from build123d import *

# Parameters (mm, degrees)
SKETCH1_W            = 82.8
SKETCH1_H            = 327.3
PCB_EXTRUDE_DEPTH    = 1.6
SKETCH2_W            = 82.8
SKETCH2_H            = 327.3
SKETCH2_W_2          = 82.5
SKETCH2_H_2          = 327
OFFSET_EDGES_DEPTH   = 10
CORNER_FILLETS_R     = 1
SKETCH3_R            = 1.5
SKETCH3_W            = 15
SKETCH3_H            = 6
SOLAR_HOLE_DEPTH     = 169.630876473
SOLAR_HOLE_FILLET_R  = 0.5
M2_CLEARANCE_HOLE1_D = 2.6
SKETCH9_W            = 1.75
SKETCH9_H            = 2.6
CUT_EXTRUDE1_DEPTH   = 169.630876473
FILLET1_R            = 2.5


with BuildPart() as part:
    # Sketch1 → PCB extrude (new body)
    with BuildSketch(Plane.XY):
        Rectangle(SKETCH1_W, SKETCH1_H)
    extrude(amount=PCB_EXTRUDE_DEPTH)

    # Sketch2 → offset edges (cut)
    with BuildSketch(Plane.XY):
        Rectangle(SKETCH2_W, SKETCH2_H)
        Rectangle(SKETCH2_W_2, SKETCH2_H_2, mode=Mode.SUBTRACT)
    extrude(amount=OFFSET_EDGES_DEPTH, mode=Mode.SUBTRACT)

    # corner fillets
    corner_fillets_edges = [part.edges().sort_by_distance(p)[0] for p in [
        (41.25, 163.5, 0.8),
        (-41.25, 163.5, 0.8),
        (-41.25, -163.5, 0.8),
        (41.25, -163.5, 0.8),
    ]]
    fillet(corner_fillets_edges, radius=CORNER_FILLETS_R)

    # Sketch3 → Solar hole (cut, symmetric)
    with BuildSketch(Plane.XY):
        with Locations((0, 160.95)):
            Circle(SKETCH3_R)
        with BuildLine():
            Line((-2.999999999, 158.15), (2.999999999, 158.15))
            Line((2.999999999, 158.15), (2.999999999, 161.65))
            Line((2.999999999, 161.65), (9.5, 161.65))
            ThreePointArc((9.5, 161.65), (10, 161.15), (9.5, 160.65))
            Line((9.5, 160.65), (6.2, 160.65))
            Line((6.2, 160.65), (6.2, 153.35))
            Line((6.2, 153.35), (-6.2, 153.35))
            Line((-6.2, 153.35), (-6.2, 160.65))
            Line((-6.2, 160.65), (-9.5, 160.65))
            ThreePointArc((-9.5, 160.65), (-10, 161.15), (-9.5, 161.65))
            Line((-9.5, 161.65), (-2.999999999, 161.65))
            Line((-2.999999999, 161.65), (-2.999999999, 158.15))
        make_face()
        with Locations((0, 42.125)):
            Rectangle(SKETCH3_W, SKETCH3_H)
    solar_hole = extrude(amount=SOLAR_HOLE_DEPTH, both=True, mode=Mode.SUBTRACT)

    # Solar hole mirror: Solar hole across plane
    add(solar_hole.mirror(Plane.ZX), mode=Mode.SUBTRACT)

    # Solar Hole Fillet
    solar_hole_fillet_edges = [part.edges().sort_by_distance(p)[0] for p in [
        (2.999999999, 161.65, 0.8),
        (2.999999999, 158.15, 0.8),
        (-2.999999999, 158.15, 0.8),
        (-2.999999999, 161.65, 0.8),
        (-6.2, 160.65, 0.8),
        (-6.2, 153.35, 0.8),
        (6.2, 153.35, 0.8),
        (6.2, 160.65, 0.8),
        (6.2, -160.65, 0.8),
        (6.2, -153.35, 0.8),
        (-6.2, -153.35, 0.8),
        (-6.2, -160.65, 0.8),
        (-2.999999999, -161.65, 0.8),
        (-2.999999999, -158.15, 0.8),
        (2.999999999, -158.15, 0.8),
        (2.999999999, -161.65, 0.8),
    ]]
    fillet(solar_hole_fillet_edges, radius=SOLAR_HOLE_FILLET_R)

    # M2 Clearance Hole1 (through all)
    with Locations(Plane.XY.offset(1.6)):
        with Locations((-39.5, 143.75), (-39.5, 113.75), (-39.5, 83.75), (-39.5, 27.25), (-39.5, 0.75), (-39.5, -25.75), (-39.5, -83.75), (-39.5, -113.75), (-39.5, -143.75), (-16.5, -117.75), (16.5, -117.75), (39.5, -143.75), (39.5, -113.75), (39.5, -83.75), (16.5, -58.1), (-16.5, -58.1), (39.5, -25.75), (39.5, 0.75), (16.5, 0), (-16.5, 0), (39.5, 27.25), (16.5, 58.1), (-16.5, 58.1), (16.5, 117.75), (-16.5, 117.75), (39.5, 83.75), (39.5, 113.75), (39.5, 143.75)):
            Hole(M2_CLEARANCE_HOLE1_D / 2)

    # Sketch9 → Cut-Extrude1 (cut, through all)
    with BuildSketch(Plane.XY):
        with Locations((-40.375, 143.75)):
            Rectangle(SKETCH9_W, SKETCH9_H)
        with Locations((40.375, 143.75)):
            Rectangle(SKETCH9_W, SKETCH9_H)
        with Locations((40.375, 113.75)):
            Rectangle(SKETCH9_W, SKETCH9_H)
        with Locations((40.375, 83.75)):
            Rectangle(SKETCH9_W, SKETCH9_H)
        with Locations((-40.375, 113.75)):
            Rectangle(SKETCH9_W, SKETCH9_H)
        with Locations((-40.375, 83.75)):
            Rectangle(SKETCH9_W, SKETCH9_H)
        with Locations((40.375, 27.25)):
            Rectangle(SKETCH9_W, SKETCH9_H)
        with Locations((-40.375, 27.25)):
            Rectangle(SKETCH9_W, SKETCH9_H)
        with Locations((40.375, 0.75)):
            Rectangle(SKETCH9_W, SKETCH9_H)
        with Locations((-40.375, 0.75)):
            Rectangle(SKETCH9_W, SKETCH9_H)
        with Locations((40.375, -25.75)):
            Rectangle(SKETCH9_W, SKETCH9_H)
        with Locations((-40.375, -25.75)):
            Rectangle(SKETCH9_W, SKETCH9_H)
        with Locations((40.375, -83.75)):
            Rectangle(SKETCH9_W, SKETCH9_H)
        with Locations((-40.375, -83.75)):
            Rectangle(SKETCH9_W, SKETCH9_H)
        with Locations((40.375, -113.75)):
            Rectangle(SKETCH9_W, SKETCH9_H)
        with Locations((-40.375, -113.75)):
            Rectangle(SKETCH9_W, SKETCH9_H)
        with Locations((40.375, -143.75)):
            Rectangle(SKETCH9_W, SKETCH9_H)
        with Locations((-40.375, -143.75)):
            Rectangle(SKETCH9_W, SKETCH9_H)
    extrude(amount=CUT_EXTRUDE1_DEPTH, mode=Mode.SUBTRACT)

    # Fillet1
    fillet1_edges = [part.edges().sort_by_distance(p)[0] for p in [
        (-7.5, -39.125, 0.8),
        (-7.5, -45.125, 0.8),
        (7.5, -45.125, 0.8),
        (7.5, -39.125, 0.8),
        (-7.5, 45.125, 0.8),
        (-7.5, 39.125, 0.8),
        (7.5, 39.125, 0.8),
        (7.5, 45.125, 0.8),
    ]]
    fillet(fillet1_edges, radius=FILLET1_R)


solid = part.part
Source: CAD feature listing. Evaluate the final solid. Frame: model axes, mm. Give positions to 0.01 mm unless a question says otherwise; leave off trailing zeros. Answer as a JSON object with one key per item and string values.
Q1. Cut plane A-A, the plane z = 0.8. Count the separate pieces of the cut face and the enclosed holes in it, then the cut area to 3 significant figures.
Geometry check:
{"separate pieces": "1", "enclosed holes": "16", "area": "26,400 mm^2"}
Q2. Ray query, line 1 along Y through (x, z) = (-16.5, 1.15); line 2 along X through (y, z) = (117.75, 0.7); line 3 along X through (y, z) = (-144, 0.95). Return the intervals inside material, ascending.
Geometry check:
{"line 1": "y = -163.5 to -119.05, -116.45 to -59.4, -56.8 to -1.3, 1.3 to 56.8, 59.4 to 116.45, 119.05 to 163.5", "line 2": "x = -41.25 to -17.8, -15.2 to 15.2, 17.8 to 41.25", "line 3": "x = -38.22 to 38.22"}
Q3. Contact query for a flat-ended pin moving along its axis: P1, Ø2.5, axis at x = 16.5, y = 0, coming from the -Z side. Output: stop coordinate, or through.
Geometry check:
{"P1": "passes through"}
